from build123d import *

# Parameters (mm, degrees)
F0_W     = 68
F0_H     = 93
F0_W_2   = 62
F0_H_2   = 87
F1_DEPTH = 3
F0_W_3   = 82
F0_H_3   = 103
F2_DEPTH = 4
F4_DEPTH = 98
F6_DEPTH = 98


with BuildPart() as f1:
    # F0 (on Top) → F1 (new body)
    with BuildSketch(Plane.XY):
        with Locations((34, 46.5)):
            Rectangle(F0_W, F0_H)
        with Locations((34, 46.5)):
            Rectangle(F0_W_2, F0_H_2, mode=Mode.SUBTRACT)
    extrude(amount=F1_DEPTH)

    # F0 (on Top) → F2 (join)
    with BuildSketch(Plane.XY):
        with Locations((34, 46.5)):
            Rectangle(F0_W_3, F0_H_3)
        with Locations((34, 46.5)):
            Rectangle(F0_W, F0_H, mode=Mode.SUBTRACT)
    extrude(amount=F2_DEPTH)

    # F3 (on Front) → F4 (join)
    with BuildSketch(Plane.XZ):
        Polygon((-5.171573, 6), (-4.171573, 4), (-1.171573, 4), (-0.171573, 6), align=None)
    extrude(amount=-F4_DEPTH)

    # F5 (on Front) → F6 (cut)
    with BuildSketch(Plane.XZ):
        Polygon((72.75, 4), (69.25, 4), (68.25, 1.499999), (73.75, 1.499999), align=None)
    extrude(amount=-F6_DEPTH, mode=Mode.SUBTRACT)


solid = f1.part
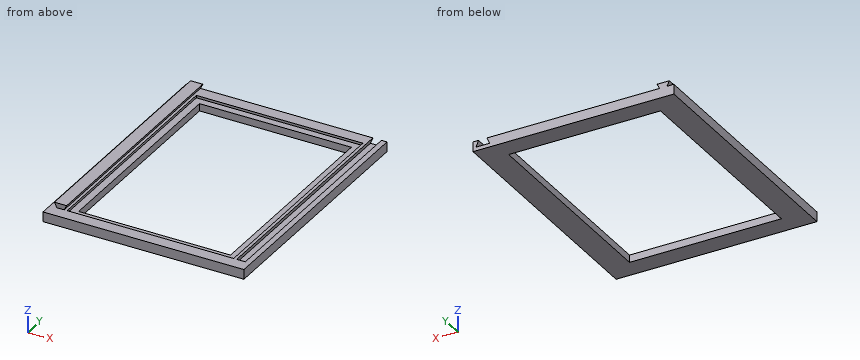
Can you work these out from the model? Positions are in its coordinate system, mm. Give positions to 0.01 mm unless a question says otherwise; leave off trailing zeros. Loops run counter-clockwise (first coordinate to the right, second up) from the corner with the lowest first, then second, coordinate; pieces in that order, holes last. Notation, with made-up numbers: (-23, -23) -> (16, -23) arc R19 ccw to (16, -17) -> close; hole circle Ø5 at (84, 1). An arc over 180 degrees is marked (long way). Return JSON: item names as keys, results as strings.
Q1. I want a section at A-A, the plane y = 51.5. List the corners of the cut face in (x, z) for me.
Checks:
{"outline": "(-7, 0) -> (3, 0) -> (3, 3) -> (0, 3) -> (0, 4) -> (-1.17, 4) -> (-0.17, 6) -> (-5.17, 6) -> (-4.17, 4) -> (-7, 4) -> close; (65, 0) -> (75, 0) -> (75, 4) -> (72.75, 4) -> (73.75, 1.5) -> (68.25, 1.5) -> (69.25, 4) -> (68, 4) -> (68, 3) -> (65, 3) -> close"}
Q2. I need wall thicknesses on probe 1 along Y at (x, z) = (61, 2.35); probe 2 along X at (y, z) = (77, 3.7); probe 3 along X at (y, z) = (41, 1.7). Which ranges of each line are inside material? Lowest first, please.
Checks:
{"probe 1": "y = -5 to 3, 90 to 98", "probe 2": "x = -7 to 0, 68 to 69.13, 72.87 to 75", "probe 3": "x = -7 to 3, 65 to 68.33, 73.67 to 75"}
Q3. I want a section at B-B, the plane x = 48.5. List the corners of the cut face in (y, z) for me, then the cut area to 3 significant figures.
Checks:
{"outline": "(-5, 0) -> (3, 0) -> (3, 3) -> (0, 3) -> (0, 4) -> (-5, 4) -> close; (90, 0) -> (98, 0) -> (98, 4) -> (93, 4) -> (93, 3) -> (90, 3) -> close", "area": "58.0 mm2"}
Q4. For pin 1 Ø1.6 at (x, y) = (70.5, 55.5) entering from +Z; pin 2 Ø1.5 at (x, y) = (3, 69) entering from +Z; pin 3 Ø1.3 at (x, z) = (71, 2.5) entering from +Y, each with a flat end and sliding along its axis, tell me the tip position at first contact or that it passes through.
Checks:
{"pin 1": "stops at z = 1.5", "pin 2": "stops at z = 3", "pin 3": "stops at y = 0"}
Q5. I want a section at C-C, the plane z = 5.1. List the corners of the cut face in (x, y) for me.
Checks:
{"outline": "(-4.72, 0) -> (-0.62, 0) -> (-0.62, 98) -> (-4.72, 98) -> close"}
